from build123d import *
from build123d.topology import SkipClean

# Parameters (mm, degrees)
SKETCH1_R                       = 12
SKETCH1_R_2                     = 1.5
SKETCH1_R_3                     = 3
BOSS_EXTRUDE1_DEPTH             = 8
SKETCH2_R                       = 5
BOSS_EXTRUDE2_DEPTH             = 4
BOSS_EXTRUDE2_DIRECTION_2_REACH = 20.762
FILLET1_R                       = 2


with BuildPart() as part:
    # Sketch1 → Boss-Extrude1 (new body)
    with BuildSketch(Plane.XY):
        Circle(SKETCH1_R)
        with Locations((0, 10)):
            Circle(SKETCH1_R_2, mode=Mode.SUBTRACT)
        Circle(SKETCH1_R_3, mode=Mode.SUBTRACT)
        with Locations((8.660254038, 5)):
            Circle(SKETCH1_R_2, mode=Mode.SUBTRACT)
        with Locations((8.660254038, -5)):
            Circle(SKETCH1_R_2, mode=Mode.SUBTRACT)
        with Locations((0, -10)):
            Circle(SKETCH1_R_2, mode=Mode.SUBTRACT)
        with Locations((-8.660254038, -5)):
            Circle(SKETCH1_R_2, mode=Mode.SUBTRACT)
        with Locations((-8.660254038, 5)):
            Circle(SKETCH1_R_2, mode=Mode.SUBTRACT)
    extrude(amount=BOSS_EXTRUDE1_DEPTH)

    # Sketch2 → Boss-Extrude2 (add)
    with SkipClean():  # the faces are left unmerged after this step: merging them gives an invalid solid
        with BuildSketch(Plane.XY.offset(8)):
            Circle(SKETCH2_R)
            with BuildLine():
                Line((1.658312395, -2.5), (-1.658312395, -2.5))
                ThreePointArc((-1.658312395, -2.5), (0, 3), (1.658312395, -2.5))
            make_face(mode=Mode.SUBTRACT)
        extrude(amount=BOSS_EXTRUDE2_DEPTH)

    # Boss-Extrude2 direction 2: up to this face of the body (flat: up to its plane)
    boss_extrude2_direction_2_end = Plane(part.part.faces().sort_by_distance((-11.660588745, 0, 0))[0])
    # Sketch2 → Boss-Extrude2 direction 2 (add, up to the picked face)
    with BuildSketch(Plane.XY.offset(8), mode=Mode.PRIVATE) as boss_extrude2_direction_2_sk1:
        Circle(SKETCH2_R)
        with BuildLine():
            Line((1.658312395, -2.5), (-1.658312395, -2.5))
            ThreePointArc((-1.658312395, -2.5), (0, 3), (1.658312395, -2.5))
        make_face(mode=Mode.SUBTRACT)
    boss_extrude2_direction_2_tool1 = split(extrude(boss_extrude2_direction_2_sk1.sketch, amount=-BOSS_EXTRUDE2_DIRECTION_2_REACH, mode=Mode.PRIVATE), bisect_by=boss_extrude2_direction_2_end, keep=Keep.BOTH, mode=Mode.PRIVATE)
    add(boss_extrude2_direction_2_tool1.solids().sort_by(Axis((-4.858579, 0, 8), (0, 0, -1)))[0])

    # Fillet1
    fillet1_edges = [part.edges().sort_by_distance(p)[0] for p in [
        (-5, 0, 8),
    ]]
    fillet(fillet1_edges, radius=FILLET1_R)


solid = part.part
Here's how the part is built. I have some questions about the finished solid (model axes, mm). A direction names the side the tool comes from. Round coordinates to 2 decimals unless told otherwise and drop trailing zeros. Write each loop counter-clockwise with the first axis right and the second up, starting at its lowest first coordinate (ties: lowest second). Pieces come first, ordered by that corner, then holes.
1. For faces 5 (the flat face through (0, -2.5, 6)), 6 (the flat face through (5.2, -5.2, 8)), 7 (the flat face through (0, -3, 12)), which set-ups out of +Z, -Z, +X, -X, +Y, -Y let a thin tool reach every point of the face, with its end or its side?
2. I need wall thicknesses on L1, parallel to Y at x = 0, z = 3; L2, parallel to Y at x = 0.5, z = 8.75; L3, parallel to Z at x = 9.5, y = 6.5. Which ranges of each line are inside material? Lowest first, please.
3. Will these pins go through, and if not, where does the flat tip stop? pin 1 Ø3.5 at (x, z) = (0.5, 3.5) entering from +Y; pin 2 Ø3 at (x, z) = (-5, 4) entering from +Y; pin 3 Ø6 at (y, z) = (4.5, 7) entering from +X.
4. Suppose I cut it at C-C (z = 11.25). List the corners of the cut face in (x, y) for me, and give its area (3 significant figures).
5. Suppose I cut it at D-D (x = -0.75). State how many separate pieces and enclosed holes the cut face has, and give its area (3 significant figures).
6. If we mould it in two halves opening along Y, with no side actions, what happens to faces 1 (the cylindrical face through (7.47, 4.09, 3.94)), 2 (the cylindrical face through (-0.325, 8.536, 3.944)), 3 (the cylindrical face through (-1.08, -4.88, 10.99)), 4 (the flat face through (2.5, -2.5, 0))? For each: released by +Y, released by -Y, zero draft, split by the parting line, or undercut.
7. Suppose I cut it at B-B (z = 1.5). List the corners of the cut face in (x, y) for me.
8. Suppose I cut it at A-A (y = 0). List the corners of the cut face in (x, z) for me.
Answer sheet:
1. face 5: +Z, -Z
1. face 6: +Z
1. face 7: +Z, +X, -X, +Y, -Y
2. L1: y = -12 to -11.5, -8.5 to -2.5, 3 to 8.5, 11.5 to 12
2. L2: y = -5.42 to -2.5, 2.96 to 5.42
2. L3: z = 0 to 8
3. pin 1: stops at y = 12
3. pin 2: stops at y = 11.48
3. pin 3: stops at x = 11.91
4. outline: circle Ø10 at (0, 0); hole (-1.66, -2.5) - (1.66, -2.5) arc R3 ccw (long way) to start
4. area: 51.4 mm2
5. separate pieces: 4
5. enclosed holes: 0
5. area: 126 mm2
6. face 1: undercut
6. face 2: undercut
6. face 3: split by the parting line
6. face 4: zero draft
7. outline: circle Ø24 at (0, 0); hole circle Ø3 at (-8.66, -5); hole circle Ø3 at (-8.66, 5); hole (-1.66, -2.5) - (1.66, -2.5) arc R3 ccw (long way) to start; hole circle Ø3 at (0, -10); hole circle Ø3 at (0, 10); hole circle Ø3 at (8.66, -5); hole circle Ø3 at (8.66, 5)
8. outline: (-12, 0) - (-3, 0) - (-3, 12) - (-5, 12) - (-5, 10) arc R2 cw to (-7, 8) - (-12, 8) - close; (3, 0) - (12, 0) - (12, 8) - (7, 8) arc R2 cw to (5, 10) - (5, 12) - (3, 12) - close
